from build123d import *

# Parameters (mm, degrees)
SKETCH1_W               = 78
SKETCH1_H               = 50
PCB_DEPTH               = 0.6
CARD_EDGES_R            = 2.54
SKETCH4_R               = 2.54
MAGNET_HOLE_CUT_DEPTH   = 93.651821353
SKETCH8_R               = 3.33
STEEL_INLAY_CUT_DEPTH   = 0.266625
MIRROR2_COPY_1_SKETCH_R = 2.54
MIRROR2_COPY_1_DEPTH    = 93.651821353
MIRROR2_COPY_2_SKETCH_R = 3.33
MIRROR2_COPY_2_DEPTH    = 0.266625
SKETCH15_R              = 10.05
BATTERY_HOLES_DEPTH     = 93.651821353


with BuildPart() as part:
    # Sketch1 → pcb (new body)
    with BuildSketch(Plane(origin=(0, 0, 0), x_dir=(1, 0, 0), z_dir=(0, 1, 0))):
        with Locations((39, 25)):
            Rectangle(SKETCH1_W, SKETCH1_H)
    extrude(amount=PCB_DEPTH)

    # card edges
    card_edges_edges = [part.edges().sort_by_distance(p)[0] for p in [
        (0, 0.3, -50),
        (78, 0.3, -50),
        (78, 0.3, 0),
        (0, 0.3, 0),
    ]]
    fillet(card_edges_edges, radius=CARD_EDGES_R)

    # Sketch4 → magnet hole cut (cut, through all)
    with BuildSketch(Plane(origin=(0, 0.6, 0), x_dir=(1, 0, 0), z_dir=(0, 1, 0))):
        with Locations(Location((4.1275, 4.13, 0), (0, 0, 270))):
            Circle(SKETCH4_R)
    magnet_hole_cut = extrude(amount=-MAGNET_HOLE_CUT_DEPTH, mode=Mode.SUBTRACT)

    # Sketch8 → steel inlay cut (cut)
    with BuildSketch(Plane.XZ):
        with Locations(Location((4.1275, -4.13, 0), (0, 0, 270))):
            Circle(SKETCH8_R)
    steel_inlay_cut = extrude(amount=-STEEL_INLAY_CUT_DEPTH, mode=Mode.SUBTRACT)

    # Mirror1: magnet hole cut, steel inlay cut across plane
    add(magnet_hole_cut.mirror(Plane.XY.offset(-25)), mode=Mode.SUBTRACT)
    add(steel_inlay_cut.mirror(Plane.XY.offset(-25)), mode=Mode.SUBTRACT)

    # Mirror2: magnet hole cut, steel inlay cut across plane
    add(magnet_hole_cut.mirror(Plane(origin=(39, 0, 0), x_dir=(0, 0, 1), z_dir=(1, 0, 0))), mode=Mode.SUBTRACT)
    add(steel_inlay_cut.mirror(Plane(origin=(39, 0, 0), x_dir=(0, 0, 1), z_dir=(1, 0, 0))), mode=Mode.SUBTRACT)

    # Mirror2 copy 1 sketch → Mirror2 copy 1 (cut, through all)
    with BuildSketch(Plane(origin=(78, 0.6, -50), x_dir=(-1, 0, 0), z_dir=(0, 1, 0))):
        with Locations(Location((4.1275, 4.13, 0), (0, 0, 270))):
            Circle(MIRROR2_COPY_1_SKETCH_R)
    extrude(amount=-MIRROR2_COPY_1_DEPTH, mode=Mode.SUBTRACT)

    # Mirror2 copy 2 sketch → Mirror2 copy 2 (cut)
    with BuildSketch(Plane(origin=(78, 0, -50), x_dir=(-1, 0, 0), z_dir=(0, -1, 0))):
        with Locations(Location((4.1275, -4.13, 0), (0, 0, 270))):
            Circle(MIRROR2_COPY_2_SKETCH_R)
    extrude(amount=-MIRROR2_COPY_2_DEPTH, mode=Mode.SUBTRACT)

    # Sketch15 → battery_holes (cut, through all)
    with BuildSketch(Plane(origin=(0, 0.6, 0), x_dir=(1, 0, 0), z_dir=(0, 1, 0))):
        with Locations(Location((61.6, 38.3625, 0), (0, 0, 270))):
            Circle(SKETCH15_R)
        with Locations(Location((39.9125, 38.3625, 0), (0, 0, 270))):
            Circle(SKETCH15_R)
    extrude(amount=-BATTERY_HOLES_DEPTH, mode=Mode.SUBTRACT)


solid = part.part
Can you work these out from the model? Positions are in its coordinate system, mm. A direction names the side the tool comes from. Coordinates: 2 decimals unless noted, no trailing zeros. Write each loop counter-clockwise with the first axis right and the second up, starting at its lowest first coordinate (ties: lowest second). Pieces come first, ordered by that corner, then holes. Notation, with made-up numbers: M 13,83.25 L 25,83.25 A37 cw 25,119.25 Z; hole C -20.5,41 d11. An arc over 180 degrees is marked long. Use one line per item in the form item = value.
Q1. We'd pull the mould along X, two halves only. Please class faces 3 (the cylindrical face through (77.276, 0.304, -49.236)), 4 (the flat face through (38, 0.6, -25)), 5 (the cylindrical face through (4.89, 0.436, -48.293)): +X half, -X half, draft (parallel to the pull), parting line (faces both ways), or undercut.
Model answer:
face_3 = +X half
face_4 = draft
face_5 = undercut
Q2. If we section it at C-C (y = 0.1): Write out the boundary of the cut face in (x, z), then the cut area to 3 significant figures.
Model answer:
outline = M 0,-47.46 A2.54 ccw 2.54,-50 L 75.46,-50 A2.54 ccw 78,-47.46 L 78,-2.54 A2.54 ccw 75.46,0 L 2.54,0 A2.54 ccw 0,-2.54 Z; hole C 4.13,-45.87 d6.66; hole C 4.13,-4.13 d6.66; hole C 39.91,-38.36 d20.1; hole C 61.6,-38.36 d20.1; hole C 73.87,-45.87 d6.66; hole C 73.87,-4.13 d6.66
area = 3,120 mm^2
Q3. For P1, Ø3, axis at x = 4.13, z = -4.13, coming from the -Y side; P2, Ø6.5, axis at x = 73.87, z = -4.13, coming from the -Y side, each with a flat end and sliding along its axis, tell me the tip position at first contact or that it passes through.
Model answer:
P1 = through
P2 = 0.27
Q4. For faces 1 (the flat face through (77, 0.267, -46)), 2 (the cylindrical face through (0.724, 0.304, -49.236)), which set-ups out of +Z, -Z, +X, -X, +Y, -Y let a thin tool reach every point of the face, with its end or its side?
Model answer:
face_1 = -Y
face_2 = -Z, -X, +Y, -Y
Q5. If we section it at A-A (z = -4.13): Write out the boundary of the cut face in (x, y), then the cut area to 3 significant figures.
Model answer:
outline = M 0,0 L 0.8,0 L 0.8,0.27 L 1.59,0.27 L 1.59,0.6 L 0,0.6 Z; M 6.67,0.27 L 7.46,0.27 L 7.46,0 L 70.54,0 L 70.54,0.27 L 71.33,0.27 L 71.33,0.6 L 6.67,0.6 Z; M 76.41,0.27 L 77.2,0.27 L 77.2,0 L 78,0 L 78,0.6 L 76.41,0.6 Z
area = 39.9 mm^2
Q6. If we section it at B-B (x = 63.5): Write out the boundary of the cut face in (y, z).
Model answer:
outline = M 0,-50 L 0.6,-50 L 0.6,-48.23 L 0,-48.23 Z; M 0,-28.49 L 0.6,-28.49 L 0.6,0 L 0,0 Z
Q7. I need wall thicknesses on line 1 along X through (y, z) = (0.2, -4.13); line 2 along Z through (x, y) = (40.5, 0.15); line 3 along X through (y, z) = (0.5, -32). Which ranges of each line are inside material? Lowest first, please. Write a range as from..to.
Model answer:
line_1 = 0..0.8, 7.46..70.54, 77.2..78
line_2 = -50..-48.4, -28.33..0
line_3 = 0..32.13, 47.69..53.82, 69.38..78
Q8. If we section it at D-D (z = -45.87): Write out the boundary of the cut face in (x, y), then the cut area to 3 significant figures.
Model answer:
outline = M 0,0 L 0.8,0 L 0.8,0.27 L 1.59,0.27 L 1.59,0.6 L 0,0.6 Z; M 6.67,0.27 L 7.46,0.27 L 7.46,0 L 33.23,0 L 33.23,0.6 L 6.67,0.6 Z; M 46.59,0 L 54.92,0 L 54.92,0.6 L 46.59,0.6 Z; M 68.28,0 L 70.54,0 L 70.54,0.27 L 71.33,0.27 L 71.33,0.6 L 68.28,0.6 Z; M 76.41,0.27 L 77.2,0.27 L 77.2,0 L 78,0 L 78,0.6 L 76.41,0.6 Z
area = 23.8 mm^2
